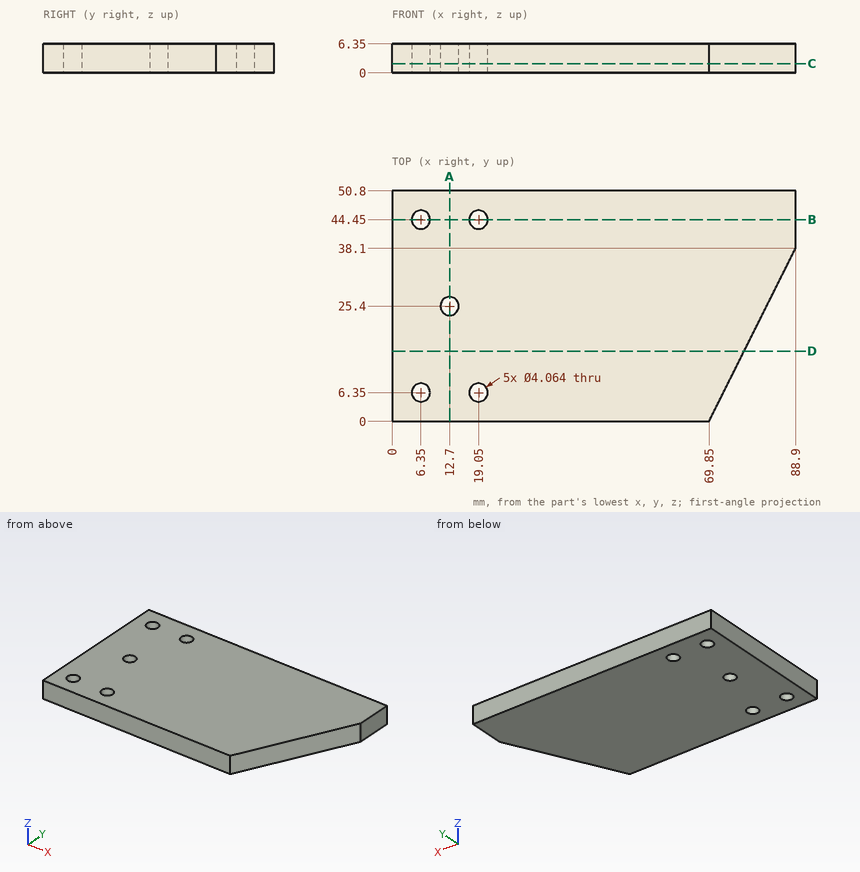
Check sheet for the drawn part. Datum: minimum x, y, z corner. Units: mm. Round coordinates to 2 decimals unless told otherwise and drop trailing zeros. Write each loop counter-clockwise with the first axis right and the second up, starting at its lowest first coordinate (ties: lowest second). Pieces come first, ordered by that corner, then holes. Notation, with made-up numbers: (76, -27) -> (131, -27) arc R23 cw to (131, -9) -> close; hole circle Ø10 at (19, 54.5). An arc over 180 degrees is marked (long way). Write each question's results on one line, items separated by ' | '.
Q1. Go/stop test with flat-tipped pins: pin 1 Ø1 at (y, z) = (23.5, 5.5) entering from +X; pin 2 Ø3 at (y, z) = (18, 2) entering from -X; pin 3 Ø1 at (y, z) = (15.5, 3) entering from +X. Record where each tip stops, or that it passes through.
Derived:
pin 1: stops at x = 81.85 | pin 2: stops at x = 0 | pin 3: stops at x = 77.85
Q2. Sectioned sample at B-B, the plane y = 44.45. Record the boundary of the cut face in (x, z), and give its area (3 significant figures).
Derived:
outline: (0, 0) -> (4.32, 0) -> (4.32, 6.35) -> (0, 6.35) -> close; (8.38, 0) -> (17.02, 0) -> (17.02, 6.35) -> (8.38, 6.35) -> close; (21.08, 0) -> (88.9, 0) -> (88.9, 6.35) -> (21.08, 6.35) -> close | area: 513 mm²
Q3. Sectioned sample at D-D, the plane y = 15.5. Record the boundary of the cut face in (x, z).
Derived:
outline: (0, 0) -> (77.6, 0) -> (77.6, 6.35) -> (0, 6.35) -> close
Q4. Sectioned sample at A-A, the plane x = 12.7. Record the boundary of the cut face in (y, z).
Derived:
outline: (0, 0) -> (23.37, 0) -> (23.37, 6.35) -> (0, 6.35) -> close; (27.43, 0) -> (50.8, 0) -> (50.8, 6.35) -> (27.43, 6.35) -> close
Q5. Sectioned sample at C-C, the plane z = 2. Record the boundary of the cut face in (x, y), and give its area (3 significant figures).
Derived:
outline: (0, 0) -> (69.85, 0) -> (88.9, 38.1) -> (88.9, 50.8) -> (0, 50.8) -> close; hole circle Ø4.06 at (6.35, 6.35); hole circle Ø4.06 at (6.35, 44.45); hole circle Ø4.06 at (12.7, 25.4); hole circle Ø4.06 at (19.05, 6.35); hole circle Ø4.06 at (19.05, 44.45) | area: 4,090 mm²
Q6. Thickness scan on probe 1 along Y at (x, z) = (19.05, 2.25); probe 2 along X at (y, z) = (7.5, 4); probe 3 along Y at (x, z) = (81.5, 6.25). Record the ranges inside material, lowest first.
Derived:
probe 1: y = 0 to 4.32, 8.38 to 42.42, 46.48 to 50.8 | probe 2: x = 0 to 4.67, 8.03 to 17.37, 20.73 to 73.6 | probe 3: y = 23.3 to 50.8
